from build123d import *

# Parameters (mm, degrees)
SKETCH1_W           = 6
SKETCH1_H           = 6
BOSS_EXTRUDE1_DEPTH = 6
SKETCH2_W           = 1.5
SKETCH2_H           = 6
BOSS_EXTRUDE2_DEPTH = 30
SKETCH3_R           = 1.5
CUT_EXTRUDE1_DEPTH  = 5


with BuildPart() as part:
    # Sketch1 → Boss-Extrude1 (new body)
    with BuildSketch(Plane(origin=(0, 0, 0), x_dir=(0, 0, -1), z_dir=(1, 0, 0))):
        Rectangle(SKETCH1_W, SKETCH1_H)
    extrude(amount=BOSS_EXTRUDE1_DEPTH)

    # Sketch2 → Boss-Extrude2 (add)
    with BuildSketch(Plane(origin=(6, 0, 0), x_dir=(0, 0, -1), z_dir=(1, 0, 0))):
        Rectangle(SKETCH2_W, SKETCH2_H)
    extrude(amount=BOSS_EXTRUDE2_DEPTH)

    # Sketch3 → Cut-Extrude1 (cut)
    with BuildSketch(Plane.ZY):
        Circle(SKETCH3_R)
    extrude(amount=-CUT_EXTRUDE1_DEPTH, mode=Mode.SUBTRACT)


solid = part.part
Geometry check sheet. Reference: the model listing, model coordinates, mm. A direction names the side the tool comes from. Coordinates: 2 decimals unless noted, no trailing zeros. Order: outer loops, then holes, each group sorted by start corner. A loop starts at its lowest first (then second) coordinate and runs counter-clockwise, first axis right, second up. Notation, with made-up numbers: (62, 17) -> (97, 17) arc R29 cw to (97, 54) -> close; hole circle Ø4 at (-26, 77.25). An arc over 180 degrees is marked (long way). Use a Markdown table: item, result. Add a question column.
1. Cross-section at C-C (x = 24). Enter the section's corners in (y, z).
2. Go/stop test with flat-tipped pins: pin 1 Ø3 at (x, y) = (23.5, -2) entering from -Z; pin 2 Ø3 at (x, y) = (13.5, 0.5) entering from +Z; pin 3 Ø1.5 at (y, z) = (0.5, 0) entering from -X; pin 4 Ø2.5 at (y, z) = (0.5, 0.5) entering from -X. Record where each tip stops, or that it passes through.
3. Set-up check for faces 1 (the face through (21, 0, 0.75)), 2 (the face through (21, 0, -0.75)), 3 (the face through (2.46, 0.07, -1.5)): record each of +Z, -Z, +X, -X, +Y, -Y from which the full face is reachable in a straight line by a thin tool's end or side.
4. Material ranges on L1, parallel to Y at x = 3.4, z = 0; L2, parallel to Z at x = 33.5, y = -0.15; L3, parallel to X at y = 2.85, z = -1.1, recorded low to high.
5. Cross-section at A-A (y = 0). Enter the section's corners in (x, z), and give its area (3 significant figures).
6. Cross-section at B-B (z = 0). Enter the section's corners in (x, y), and give its area (3 significant figures).
7. Cross-section at D-D (y = -1.85). Enter the section's corners in (x, z).
8. Mould release check, pull along Y, two halves, no side actions. Record for faces 4 (the face through (14, -3, 0)), 5 (the face through (6, 0, 2)), 6 (the face through (5, 0, 0)): pulls with the +Y half, pulls with the -Y half, needs draft (parallel to the pull), parting line crosses it, or undercut.
Filled sheet:
| question | item | result |
|---|---|---|
| 1 | outline | (-3, -0.75) -> (3, -0.75) -> (3, 0.75) -> (-3, 0.75) -> close |
| 2 | pin 1 | z = -0.75 |
| 2 | pin 2 | z = 0.75 |
| 2 | pin 3 | x = 5 |
| 2 | pin 4 | x = 0 |
| 3 | face 1 | +Z, +X, +Y, -Y |
| 3 | face 2 | -Z, +X, +Y, -Y |
| 3 | face 3 | -X |
| 4 | L1 | -3 to -1.5, 1.5 to 3 |
| 4 | L2 | -0.75 to 0.75 |
| 4 | L3 | 0 to 6 |
| 5 | outline | (0, -3) -> (6, -3) -> (6, -0.75) -> (36, -0.75) -> (36, 0.75) -> (6, 0.75) -> (6, 3) -> (0, 3) -> (0, 1.5) -> (5, 1.5) -> (5, -1.5) -> (0, -1.5) -> close |
| 5 | area | 66.0 mm2 |
| 6 | outline | (0, -3) -> (36, -3) -> (36, 3) -> (0, 3) -> (0, 1.5) -> (5, 1.5) -> (5, -1.5) -> (0, -1.5) -> close |
| 6 | area | 201 mm2 |
| 7 | outline | (0, -3) -> (6, -3) -> (6, -0.75) -> (36, -0.75) -> (36, 0.75) -> (6, 0.75) -> (6, 3) -> (0, 3) -> close |
| 8 | face 4 | pulls with the -Y half |
| 8 | face 5 | needs draft |
| 8 | face 6 | undercut |
